```python
from build123d import *

# Parameters (mm, degrees)
CYLINDER022_R     = 1
CYLINDER022_DEPTH = 10
CYLINDER023_R     = 1
CYLINDER023_DEPTH = 10
CYLINDER021_R     = 11.3
CYLINDER021_DEPTH = 16
CYLINDER020_R     = 7.3
CYLINDER020_DEPTH = 15
CYLINDER007_R     = 7.3
CYLINDER007_DEPTH = 15
CYLINDER019_R     = 7.3
CYLINDER019_DEPTH = 52
PAD002_DEPTH      = 4


with BuildPart() as cilindro007:
    # Cylinder022 → Cylinder022 (new body)
    with BuildSketch(Plane(origin=(-28, 0, -4), x_dir=(1, 0, 0), z_dir=(0, 0, 1))):
        Circle(CYLINDER022_R)
    extrude(amount=CYLINDER022_DEPTH)


with BuildPart() as fusion001013:
    # Cylinder023 → Cylinder023 (new body)
    with BuildSketch(Plane(origin=(-56, 0, -4), x_dir=(1, 0, 0), z_dir=(0, 0, 1))):
        Circle(CYLINDER023_R)
    extrude(amount=CYLINDER023_DEPTH)

    # Fusion001013: union Cilindro007
    add(cilindro007.part)


with BuildPart() as fusion001013_1:
    # Fusion001013 placement: moved
    add(fusion001013.part.moved(Location((0, 0, 27))))


with BuildPart() as eje004:
    # Cylinder021 → Cylinder021 (new body)
    with BuildSketch(Plane.XY.offset(15)):
        Circle(CYLINDER021_R)
    extrude(amount=CYLINDER021_DEPTH)


with BuildPart() as eje003:
    # Cylinder020 → Cylinder020 (new body)
    with BuildSketch(Plane(origin=(-28, 0, 13), x_dir=(1, 0, 0), z_dir=(0, 0, 1))):
        Circle(CYLINDER020_R)
    extrude(amount=CYLINDER020_DEPTH)


with BuildPart() as fusion001011:
    # Cylinder007 → Cylinder007 (new body)
    with BuildSketch(Plane(origin=(-56, 0, 13), x_dir=(1, 0, 0), z_dir=(0, 0, 1))):
        Circle(CYLINDER007_R)
    extrude(amount=CYLINDER007_DEPTH)

    # Fusion001011: union Eje003
    add(eje003.part)


with BuildPart() as eje001:
    # Cylinder019 → Cylinder019 (new body)
    with BuildSketch(Plane(origin=(-84, 0, -24), x_dir=(1, 0, 0), z_dir=(0, 0, 1))):
        Circle(CYLINDER019_R)
    extrude(amount=CYLINDER019_DEPTH)


with BuildPart() as cut010002:
    # Sketch004 → Pad002 (new body)
    with BuildSketch(Plane.XY):
        with BuildLine():
            Line((0, 17.7), (-83.4, 17.7))
            ThreePointArc((-83.4, 17.7), (-101.1, 0), (-83.4, -17.7))
            Line((0, -17.7), (-83.4, -17.7))
            Line((0, 17.7), (0, -17.7))
        make_face()
    extrude(amount=PAD002_DEPTH)


with BuildPart() as cut010002_1:
    # Body005 placement: moved
    add(cut010002.part.moved(Location((0, 0, 26))))

    # Cut: cut Eje001
    add(eje001.part, mode=Mode.SUBTRACT)

    # Cut026: cut Fusion001011
    add(fusion001011.part, mode=Mode.SUBTRACT)

    # Cut027: cut Eje004
    add(eje004.part, mode=Mode.SUBTRACT)

    # Cut010002: cut Fusion001013
    add(fusion001013_1.part, mode=Mode.SUBTRACT)


with BuildPart() as obj1:
    # Part__Mirroring011: instance of Cut010002
    add(cut010002_1.part.mirror(Plane(origin=(0, 0, 0), x_dir=(0, -1, 0), z_dir=(1, 0, 0))))


solid = obj1.part
```
Can you work these out from the model? Positions are in its coordinate system, mm. A direction names the side the tool comes from. Round coordinates to 2 decimals unless told otherwise and drop trailing zeros. Loops run counter-clockwise (first coordinate to the right, second up) from the corner with the lowest first, then second, coordinate; pieces in that order, holes last. Notation, with made-up numbers: M 57.5,-8 L 62.5,-8 A23 cw 62.5,3 Z; hole C 2,87 d7. An arc over 180 degrees is marked long. Write item = value, one per line. Start each with the question number.
(1) If we mould it in two halves opening along X, with no side actions, what happens to faces 3 (the face through (0, -14, 28)), 4 (the face through (56, -2, 28)), 5 (the face through (35.293, 0.321, 26.986)), 6 (the face through (41, -17.7, 28))? For each: released by +X, released by -X, zero draft, split by the parting line, or undercut.
(2) Suppose I cut it at C-C on z = 28.7. Write out the boundary of the cut face in (x, y).
(3) Suppose I cut it at A-A on x = 28. Write out the boundary of the cut face in (y, z), plus the area to 3 significant figures.
(4) Suppose I cut it at D-D on y = 4.5. Write out the boundary of the cut face in (x, z), plus the area to 3 significant figures.
(5) I need wall thicknesses on line 1 along X through (y, z) = (0, 29.2); line 2 along X through (y, z) = (0, 26.7); line 3 along Y through (x, z) = (56, 29.1). Which ranges of each line are inside material? Lowest first, please.
(6) I'm going to push flat-ended pins straight in: P1, Ø7.5, axis at x = 84, y = -2, coming from the -Z side; P2, Ø1.2, axis at x = 56, y = 0, coming from the +Z side; P3, Ø1, axis at y = -9.5, z = 29.5, coming from the +X side; P4, Ø1.5, axis at y = 11, z = 27, coming from the +X side. Where does each tip first touch, or does it pass through?
(7) Suppose I cut it at B-B on y = 0. Write out the boundary of the cut face in (x, z).
(8) Which directions (+Z, -Z, +X, -X, +Y, -Y) give clear straight access to the entire face, cutting with the end or side of a thin tool? Please do faces 1 (the face through (41, 17.7, 28)), 2 (the face through (63.293, 0.321, 26.986)).
Answer block:
q1.face_3 = released by -X
q1.face_4 = undercut
q1.face_5 = undercut
q1.face_6 = zero draft
q2.outline = M 0,-17.7 L 83.4,-17.7 A17.7 ccw 83.4,17.7 L 0,17.7 L 0,11.3 A11.3 cw 0,-11.3 Z; hole C 28,0 d2; hole C 56,0 d2
q3.outline = M -17.7,26 L -7.3,26 L -7.3,28 L -1,28 L -1,30 L -17.7,30 Z; M 1,28 L 7.3,28 L 7.3,26 L 17.7,26 L 17.7,30 L 1,30 Z
q3.area = 108 mm²
q4.outline = M 10.37,26 L 22.25,26 L 22.25,28 L 33.75,28 L 33.75,26 L 50.25,26 L 50.25,28 L 61.75,28 L 61.75,26 L 78.25,26 L 78.25,28 L 89.75,28 L 89.75,26 L 100.52,26 L 100.52,30 L 10.37,30 Z
q4.area = 292 mm²
q5.line_1 = 11.3 to 27, 29 to 55, 57 to 101.1
q5.line_2 = 11.3 to 20.7, 35.3 to 48.7, 63.3 to 76.7, 91.3 to 101.1
q5.line_3 = -17.7 to -1, 1 to 17.7
q6.P1 = 28
q6.P2 = through
q6.P3 = 98.64
q6.P4 = 97.83
q7.outline = M 11.3,26 L 20.7,26 L 20.7,28 L 27,28 L 27,30 L 11.3,30 Z; M 29,28 L 35.3,28 L 35.3,26 L 48.7,26 L 48.7,28 L 55,28 L 55,30 L 29,30 Z; M 57,28 L 63.3,28 L 63.3,26 L 76.7,26 L 76.7,28 L 91.3,28 L 91.3,26 L 101.1,26 L 101.1,30 L 57,30 Z
q8.face_1 = +Z, -Z, +X, -X, +Y
q8.face_2 = -Z
